Source: three-view drawing plus pictorial views. Frame: mm from the lowest corner of the part. A direction names the side the tool comes from. Give positions to 0.01 mm unless a question says otherwise; leave off trailing zeros. Loops run counter-clockwise (first coordinate to the right, second up) from the corner with the lowest first, then second, coordinate; pieces in that order, holes last. Notation, with made-up numbers: (86.25, 22.25) - (91.25, 22.25) arc R13 ccw to (91.25, 28.25) - close; hole circle Ø7 at (-18.75, -34.5). An arc over 180 degrees is marked (long way). Write each question's results on one line, items separated by ' | '. Start each with the question number.
(1) Reachability of the marked faces 1, 2 and 3 from +Z, -Z, +X, -X, +Y, -Y: full face, straight path, thin tool, end or side. Return the list, or none.
(2) Cut plane C-C on z = 36. Return the cut outline in (x, y).
(3) Contact query for flat-ended pins moving along their axis: pin 1 (6 mm diameter, centred on y = 3, z = 9, fed in from -X); pin 2 (1 mm diameter, centred on x = 11, z = 56.5, fed in from +Y) (1 decimal); pin 3 (2.5 mm diameter, centred on x = 7.25, y = 7.25, fed in from -Z); pin 4 (1 mm diameter, centred on x = 7.5, z = 23.5, fed in from -Y). Output: stop coordinate, or through.
(4) Cut plane A-A on x = 7.25. Return the cut outline in (y, z), then the cut area to 3 significant figures.
(5) Material intervals for line 1 along X through (y, z) = (7.25, 44); line 2 along Y through (x, z) = (7.25, 20.5), sorted ascending. Write a range as [from, to].
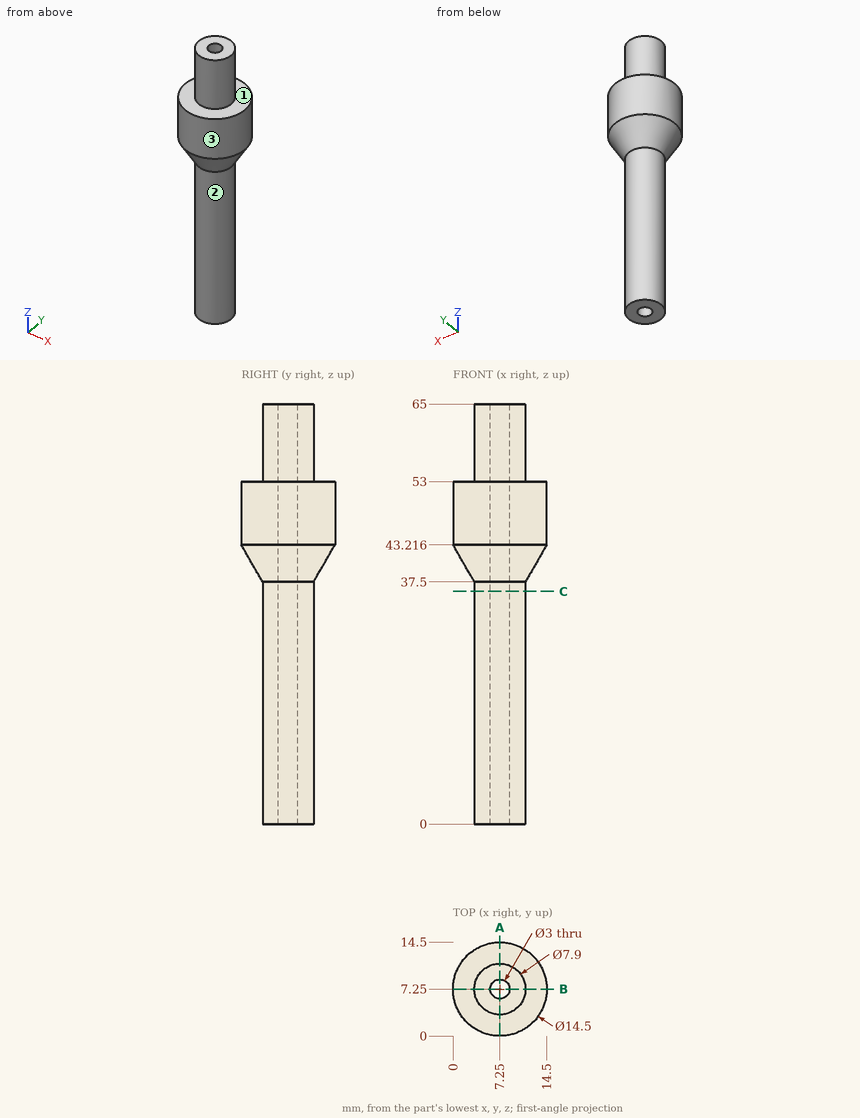
Ans:
1) face 1: +Z | face 2: -Z | face 3: +Z, -Z
2) outline: circle Ø7.9 at (7.25, 7.25); hole circle Ø3 at (7.25, 7.25)
3) pin 1: x = 3.5 | pin 2: y = 9.5 | pin 3: through | pin 4: y = 3.3
4) outline: (0, 43.22) - (3.3, 37.5) - (3.3, 0) - (5.75, 0) - (5.75, 65) - (3.3, 65) - (3.3, 53) - (0, 53) - close; (8.75, 0) - (11.2, 0) - (11.2, 37.5) - (14.5, 43.22) - (14.5, 53) - (11.2, 53) - (11.2, 65) - (8.75, 65) - close | area: 402 mm^2
5) line 1: [0, 5.75], [8.75, 14.5] | line 2: [3.3, 5.75], [8.75, 11.2]
